from build123d import *

# Parameters (mm, degrees)
SKETCH_1_R      = 3.5
EXTRUDE_1_DEPTH = 2.3
SKETCH_3_W      = 15
SKETCH_3_H      = 2.3


with BuildPart() as part:
    # 草图1 → 凸台-拉伸1 (new body)
    with BuildSketch(Plane.XY):
        with BuildLine():
            Line((-12.231269749, -8.683089331), (-6.66916341, -26.126560465))
            ThreePointArc((-6.66916341, -26.126560465), (0, -31), (6.66916341, -26.126560465))
            Line((6.66916341, -26.126560465), (12.231269749, -8.683089331))
            ThreePointArc((12.231269749, -8.683089331), (15, 0), (12.231269749, 8.683089331))
            Line((12.231269749, 8.683089331), (6.66916341, 26.126560465))
            ThreePointArc((6.66916341, 26.126560465), (0, 31), (-6.66916341, 26.126560465))
            Line((-6.66916341, 26.126560465), (-12.231269749, 8.683089331))
            ThreePointArc((-12.231269749, 8.683089331), (-15, 0), (-12.231269749, -8.683089331))
        make_face()
        with Locations((0, -24)):
            Circle(SKETCH_1_R, mode=Mode.SUBTRACT)
        with Locations((0, 24)):
            Circle(SKETCH_1_R, mode=Mode.SUBTRACT)
    extrude(amount=EXTRUDE_1_DEPTH)

    # 草图2 → 旋转1 (revolve)
    with BuildSketch(Plane(origin=(0, 0, 0), x_dir=(1, 0, 0), z_dir=(0, 1, 0)), mode=Mode.PRIVATE) as revolve_1_sk:
        Polygon((0, -2.3), (15, -2.3), (12.5, -3.8), (12.5, -14.2), (15, -15.7), (0, -15.7), align=None)
    revolve(revolve_1_sk.sketch.rotate(Axis((0, 0, 15.7), (0, 0, -1)), 180), axis=Axis((0, 0, 15.7), (0, 0, -1)))

    # 草图3 → 旋转2 (revolve)
    with BuildSketch(Plane(origin=(0, 0, 0), x_dir=(1, 0, 0), z_dir=(0, 1, 0)), mode=Mode.PRIVATE) as revolve_2_sk:
        with Locations((7.5, -16.85)):
            Rectangle(SKETCH_3_W, SKETCH_3_H)
    revolve(revolve_2_sk.sketch.rotate(Axis((0, 0, 18), (0, 0, -1)), 180), axis=Axis((0, 0, 18), (0, 0, -1)))

    # 草图4 → 切除-旋转1 (revolve, cut)
    with BuildSketch(Plane(origin=(0, 0, 0), x_dir=(1, 0, 0), z_dir=(0, 1, 0)), mode=Mode.PRIVATE) as cut_revolve_1_sk:
        Polygon((0, -10.8), (4, -10.8), (3.233, -11.3), (3.233, -18), (0, -18), align=None)
    revolve(cut_revolve_1_sk.sketch.rotate(Axis((0, 0, 18), (0, 0, -1)), 180), axis=Axis((0, 0, 18), (0, 0, -1)), mode=Mode.SUBTRACT)


solid = part.part
Can you work these out from the model? Positions are in its coordinate system, mm. A direction names the side the tool comes from. Give positions to 0.01 mm unless a question says otherwise; leave off trailing zeros. Order: outer loops, then holes, each group sorted by start corner. A loop starts at its lowest first (then second) coordinate and runs counter-clockwise, first axis right, second up. Notation, with made-up numbers: M 1.25,54.25 L 34.25,54.25 A18 ccw 34.25,75.25 Z; hole C -5,59.5 d5. An arc over 180 degrees is marked long. One line per item, written item: value.
Item 1: If we section it at B-B on y = -24: Write out the boundary of the cut face in (x, z).
Verdict:
outline: M -7.35,0 L -3.5,0 L -3.5,2.3 L -7.35,2.3 Z; M 3.5,0 L 7.35,0 L 7.35,2.3 L 3.5,2.3 Z
Item 2: If we section it at D-D on y = 0: Write out the boundary of the cut face in (x, z), and give its area (3 significant figures).
Verdict:
outline: M -15,0 L 15,0 L 15,2.3 L 12.5,3.8 L 12.5,14.2 L 15,15.7 L 15,18 L 3.23,18 L 3.23,11.3 L 4,10.8 L -4,10.8 L -3.23,11.3 L -3.23,18 L -15,18 L -15,15.7 L -12.5,14.2 L -12.5,3.8 L -15,2.3 Z
area: 434 mm2
Item 3: Please list where these lines run through material, in increasing order: line 1 (Y direction, x = 0, z = 0.95); line 2 (Z direction, x = -7.5, y = 19); line 3 (Y direction, x = 0, z = 16).
Verdict:
line 1: -31 to -27.5, -20.5 to 20.5, 27.5 to 31
line 2: 0 to 2.3
line 3: -15 to -3.23, 3.23 to 15
Item 4: For pin 1 (5 mm diameter, centred on y = -17, z = 6.5, fed in from -X); pin 2 (1.5 mm diameter, centred on y = -24, z = 2.5, fed in from +X); pin 3 (6 mm diameter, centred on x = 0, y = 0, fed in from -Z); pin 4 (5 mm diameter, centred on x = -5.5, z = 6, fed in from -Y), each with a flat end and sliding along its axis, tell me the tip position at first contact or that it passes through.
Verdict:
pin 1: through
pin 2: x = 7.58
pin 3: z = 0
pin 4: y = -12.13
Item 5: If we section it at C-C on z = 12.25: Write out the boundary of the cut face in (x, y).
Verdict:
outline: C 0,0 d25; hole C 0,0 d6.47
Item 6: If we section it at A-A on x = 0: Write out the boundary of the cut face in (y, z).
Verdict:
outline: M -31,0 L -27.5,0 L -27.5,2.3 L -31,2.3 Z; M -20.5,0 L 20.5,0 L 20.5,2.3 L 15,2.3 L 12.5,3.8 L 12.5,14.2 L 15,15.7 L 15,18 L 3.23,18 L 3.23,11.3 L 4,10.8 L -4,10.8 L -3.23,11.3 L -3.23,18 L -15,18 L -15,15.7 L -12.5,14.2 L -12.5,3.8 L -15,2.3 L -20.5,2.3 Z; M 27.5,0 L 31,0 L 31,2.3 L 27.5,2.3 Z
Item 7: If we mould it in two halves opening along Y, with no side actions, what happens to faces 4 (the face through (0, 31, 1)), 5 (the face through (-0.46, -20.53, 1.13)), 6 (the face through (-5.84, -11.228, 14.294))? For each: pulls with the +Y half, pulls with the -Y half, needs draft (parallel to the pull), parting line crosses it, or undercut.
Verdict:
face 4: pulls with the +Y half
face 5: undercut
face 6: parting line crosses it
Item 8: For faces 1 (the face through (-8.06, 12.65, 16.83)), 2 (the face through (-11.923, 3.755, 9.073)), 3 (the face through (9.41, -17.53, 1.13)), which set-ups out of +Z, -Z, +X, -X, +Y, -Y let a thin tool reach every point of the face, with its end or its side?
Verdict:
face 1: +Z
face 2: none
face 3: +Z, -Z, +X, -Y
